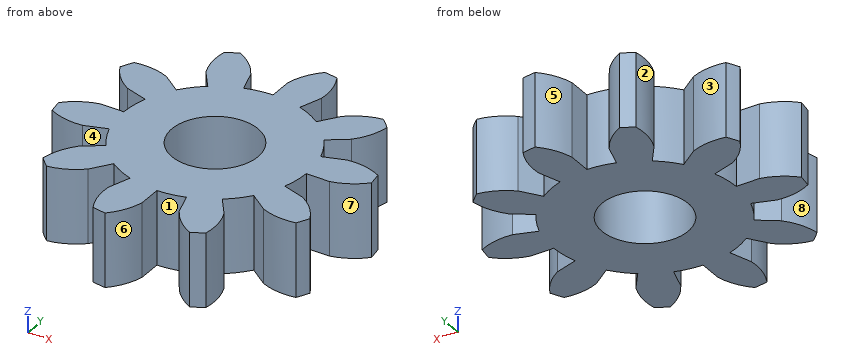
```python
from build123d import *

# Parameters (mm, degrees)
BOSS_EXTRU_1_DEPTH           = 3
R_P_TITION_CIRCULAIRE2_COUNT = 10
ESQUISSE5_R                  = 3.75
BOSS_EXTRU_2_DEPTH           = 3
ESQUISSE6_R                  = 1.75
ENL_V_MAT_EXTRU_1_DEPTH      = 4


with BuildPart() as part:
    # Esquisse4 → Boss.-Extru.1 (new body)
    with BuildSketch(Plane.XY):
        with BuildLine():
            Line((0, 4.698463104), (0, 3.75))
            ThreePointArc((0, 3.75), (0.618511546, 3.69864076), (1.220081074, 3.54596985))
            Line((1.220081074, 3.54596985), (1.528668242, 4.442828935))
            ThreePointArc((1.528668242, 4.442828935), (1.503976571, 5.174164178), (1.263823322, 5.865385802))
            ThreePointArc((1.263823322, 5.865385802), (0.989618473, 5.917825215), (0.71327115, 5.957452834))
            ThreePointArc((0.71327115, 5.957452834), (0.261291789, 5.381974273), (0, 4.698463104))
        make_face()
    extrude(amount=BOSS_EXTRU_1_DEPTH)


with BuildPart() as r_p_tition_circulaire2_1:
    # R_p_tition circulaire2: pattern copy
    add(part.part.rotate(Axis((0, 0, 0), (0, 0, 1)), 1 * 360 / R_P_TITION_CIRCULAIRE2_COUNT))


with BuildPart() as r_p_tition_circulaire2_2:
    # R_p_tition circulaire2: pattern copy
    add(part.part.rotate(Axis((0, 0, 0), (0, 0, 1)), 2 * 360 / R_P_TITION_CIRCULAIRE2_COUNT))


with BuildPart() as r_p_tition_circulaire2_3:
    # R_p_tition circulaire2: pattern copy
    add(part.part.rotate(Axis((0, 0, 0), (0, 0, 1)), 3 * 360 / R_P_TITION_CIRCULAIRE2_COUNT))


with BuildPart() as r_p_tition_circulaire2_4:
    # R_p_tition circulaire2: pattern copy
    add(part.part.rotate(Axis((0, 0, 0), (0, 0, 1)), 4 * 360 / R_P_TITION_CIRCULAIRE2_COUNT))


with BuildPart() as r_p_tition_circulaire2_5:
    # R_p_tition circulaire2: pattern copy
    add(part.part.rotate(Axis((0, 0, 0), (0, 0, 1)), 5 * 360 / R_P_TITION_CIRCULAIRE2_COUNT))


with BuildPart() as r_p_tition_circulaire2_6:
    # R_p_tition circulaire2: pattern copy
    add(part.part.rotate(Axis((0, 0, 0), (0, 0, 1)), 6 * 360 / R_P_TITION_CIRCULAIRE2_COUNT))


with BuildPart() as r_p_tition_circulaire2_7:
    # R_p_tition circulaire2: pattern copy
    add(part.part.rotate(Axis((0, 0, 0), (0, 0, 1)), 7 * 360 / R_P_TITION_CIRCULAIRE2_COUNT))


with BuildPart() as r_p_tition_circulaire2_8:
    # R_p_tition circulaire2: pattern copy
    add(part.part.rotate(Axis((0, 0, 0), (0, 0, 1)), 8 * 360 / R_P_TITION_CIRCULAIRE2_COUNT))


with BuildPart() as r_p_tition_circulaire2_9:
    # R_p_tition circulaire2: pattern copy
    add(part.part.rotate(Axis((0, 0, 0), (0, 0, 1)), 9 * 360 / R_P_TITION_CIRCULAIRE2_COUNT))


with BuildPart() as part_1:
    add(part.part)

    add(r_p_tition_circulaire2_1.part)  # Boss.-Extru.2 merges R_p_tition circulaire2_1

    add(r_p_tition_circulaire2_2.part)  # Boss.-Extru.2 merges R_p_tition circulaire2_2

    add(r_p_tition_circulaire2_3.part)  # Boss.-Extru.2 merges R_p_tition circulaire2_3

    add(r_p_tition_circulaire2_4.part)  # Boss.-Extru.2 merges R_p_tition circulaire2_4

    add(r_p_tition_circulaire2_5.part)  # Boss.-Extru.2 merges R_p_tition circulaire2_5

    add(r_p_tition_circulaire2_6.part)  # Boss.-Extru.2 merges R_p_tition circulaire2_6

    add(r_p_tition_circulaire2_7.part)  # Boss.-Extru.2 merges R_p_tition circulaire2_7

    add(r_p_tition_circulaire2_8.part)  # Boss.-Extru.2 merges R_p_tition circulaire2_8

    add(r_p_tition_circulaire2_9.part)  # Boss.-Extru.2 merges R_p_tition circulaire2_9
    # Esquisse5 → Boss.-Extru.2 (add)
    with BuildSketch(Plane.XY):
        Circle(ESQUISSE5_R)
    extrude(amount=BOSS_EXTRU_2_DEPTH)

    # Esquisse6 → Enl_v. mat.-Extru.1 (cut, through all)
    with BuildSketch(Plane.XY.offset(3)):
        Circle(ESQUISSE6_R)
    extrude(amount=-ENL_V_MAT_EXTRU_1_DEPTH, mode=Mode.SUBTRACT)


solid = part_1.part
```
Check sheet for the modelled part. Datum: model origin and axes. Units: mm. Face numbers are marked on the shaded views. A direction names the side the tool comes from. Coordinates: 2 decimals unless noted, no trailing zeros. Order: outer loops, then holes, each group sorted by start corner. A loop starts at its lowest first (then second) coordinate and runs counter-clockwise, first axis right, second up. Notation, with made-up numbers: M 17.5,73 L 35.5,73 A27 ccw 35.5,99 Z; hole C 30.25,-36.5 d9. An arc over 180 degrees is marked long. Write each question's results on one line, items separated by ' | '. Start each with the question number.
1. Cross-section at B-B on y = 1. Record the cut outline in (x, z).
2. Cross-section at A-A on x = 0.5. Record the cut outline in (y, z), and give its area (3 significant figures).
3. Go/stop test with flat-tipped pins: P1, Ø2, axis at x = 0, y = 0, coming from the +Z side; P2, Ø1.5, axis at y = 2.5, z = 1, coming from the +X side; P3, Ø1.5, axis at x = 0, y = -2.5, coming from the -Z side; P4, Ø1, axis at y = -2.5, z = 2.5, coming from the +X side. Record where each tip stops, or that it passes through.
4. Material ranges on probe 1 along X at (y, z) = (-5, 1.4); probe 2 along X at (y, z) = (-1, 2.6); probe 3 along Y at (x, z) = (0.5, 0.65), recorded low to high.
5. Access from +Z, -Z, +X, -X, +Y, -Y to the whole of each face (thin tool, end or side, straight path). Record for the marked faces 5, 6, 7 and 8.
6. Mould release check, pull along Y, two halves, no side actions. Record for the marked faces 1, 2, 3 and 4: +Y half, -Y half, draft (parallel to the pull), parting line (faces both ways), or undercut.
Checks:
1) outline: M -3.61,0 L -1.44,0 L -1.44,3 L -3.61,3 Z; M 1.44,0 L 5.92,0 L 5.92,3 L 1.44,3 Z
2) outline: M -3.72,0 L -1.68,0 L -1.68,3 L -3.72,3 Z; M 1.68,0 L 5.73,0 L 5.73,3 L 1.68,3 Z | area: 18.3 mm²
3) P1: passes through | P2: stops at x = 4.23 | P3: stops at z = 0 | P4: stops at x = 5.45
4) probe 1: x = -1.53 to -0.09, 1.75 to 2.96 | probe 2: x = -5.92 to -1.44, 1.44 to 3.61 | probe 3: y = -3.72 to -1.68, 1.68 to 5.73
5) face 5: +Z, -Z, +Y | face 6: +Z, -Z, -Y | face 7: +Z, -Z, +X | face 8: +Z, -Z, -X
6) face 1: -Y half | face 2: undercut | face 3: +Y half | face 4: undercut
